Verification items for this drawing (mm, ordinates from the low corner). Give positions to 0.01 mm unless a question says otherwise; leave off trailing zeros. Order: outer loops, then holes, each group sorted by start corner. A loop starts at its lowest first (then second) coordinate and runs counter-clockwise, first axis right, second up. Notation, with made-up numbers: (71.25, -4.75) -> (92.25, -4.75) arc R18 ccw to (92.25, 21.25) -> close; hole circle Ø8 at (68.5, 36). An arc over 180 degrees is marked (long way). One line per question, with ' | ' between items.
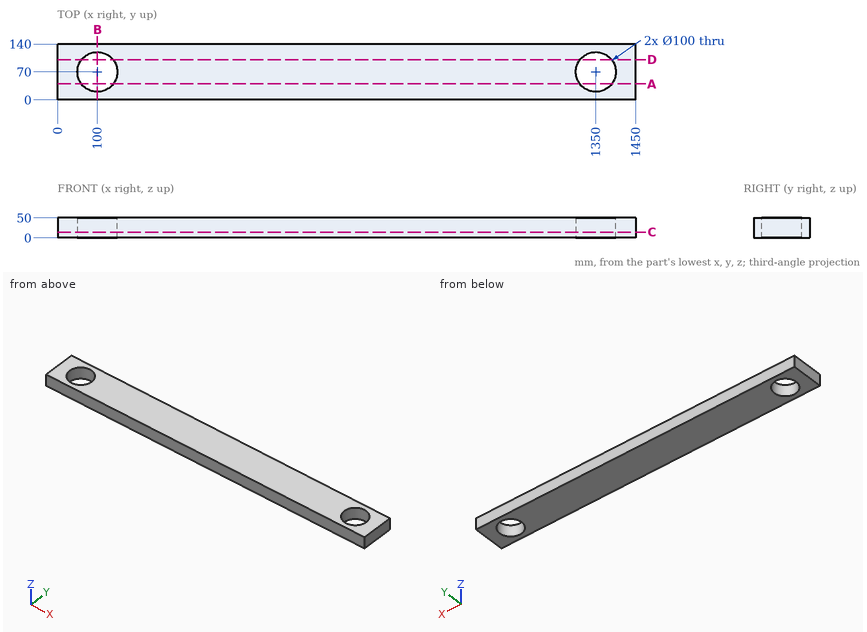
Q1. Depth check by flat-ended pin: pin 1 Ø6 at (y, z) = (15.5, 14) entering from -X. Enter the tip coordinate at first touch or a pass-through.
Result sheet:
pin 1: stops at x = 0
Q2. Section check C-C (z = 14). Enter the section's corners in (x, y), and give its area (3 significant figures).
Result sheet:
outline: (0, 0) -> (1450, 0) -> (1450, 140) -> (0, 140) -> close; hole circle Ø100 at (100, 70); hole circle Ø100 at (1350, 70) | area: 187,000 mm2
Q3. Thickness scan on line 1 (Y direction, x = 100, z = 13.5); line 2 (X direction, y = 86, z = 14); line 3 (X direction, y = 42.5, z = 2). Record the ranges inside material, lowest first.
Result sheet:
line 1: y = 0 to 20, 120 to 140 | line 2: x = 0 to 52.63, 147.37 to 1302.63, 1397.37 to 1450 | line 3: x = 0 to 58.24, 141.76 to 1308.24, 1391.76 to 1450
Q4. Section check A-A (y = 40). Enter the section's corners in (x, z).
Result sheet:
outline: (0, 0) -> (60, 0) -> (60, 50) -> (0, 50) -> close; (140, 0) -> (1310, 0) -> (1310, 50) -> (140, 50) -> close; (1390, 0) -> (1450, 0) -> (1450, 50) -> (1390, 50) -> close
Q5. Section check D-D (y = 101). Enter the section's corners in (x, z).
Result sheet:
outline: (0, 0) -> (60.77, 0) -> (60.77, 50) -> (0, 50) -> close; (139.23, 0) -> (1310.77, 0) -> (1310.77, 50) -> (139.23, 50) -> close; (1389.23, 0) -> (1450, 0) -> (1450, 50) -> (1389.23, 50) -> close
Q6. Section check B-B (x = 100). Enter the section's corners in (y, z).
Result sheet:
outline: (0, 0) -> (20, 0) -> (20, 50) -> (0, 50) -> close; (120, 0) -> (140, 0) -> (140, 50) -> (120, 50) -> close
